The listing builds one solid part. Answer for the finished solid, in the listing's coordinates (mm). A direction names the side the tool comes from. Give positions to 0.01 mm unless a question says otherwise; leave off trailing zeros. Loops run counter-clockwise (first coordinate to the right, second up) from the corner with the lowest first, then second, coordinate; pieces in that order, holes last. Notation, with made-up numbers: (-8, 10.5) - (44, 10.5) arc R10 cw to (44, 22.5) - close; hole circle Ø10 at (-40, -21.5). An arc over 180 degrees is marked (long way). Write item = value, one per line. Start each with the question number.
1) The part is cut by section B-B on y = 30. State how many separate pieces and enclosed holes the cut face has, plus the area to 3 significant figures.
2) The part is cut by section C-C on x = 2.25. Write down the section's boundary in (y, z), plus the area to 3 significant figures.
3) Consider probe 1 along Z at (x, y) = (11.6, 0); probe 2 along X at (y, z) = (-15.5, 25); probe 3 along X at (y, z) = (-11, 26). Determine where each line is inside the solid, lowest interval first.
4) The mould has two halves that part along Z. Classify faces 1 (the conical face through (8.09, -25.76, 3.38)), 2 (the flat face through (14, -0.2, 10.4)), 3 (the flat face through (9, 5, -16)): +Z half, -Z half, draft (parallel to the pull), parting line (faces both ways), or undercut.
5) Flat-ended cylindrical pins translate along their axes: P1, Ø11.5, axis at y = 0, z = 0, coming from the +X side; P2, Ø1, axis at x = 1, y = 13, coming from the +Z side; P3, Ø3.5, axis at x = -0.5, y = 10.5, coming from the -Z side; P4, Ø12, axis at x = 3.5, z = 22, coming from the -Y side. Find the tip coordinate at first contact, or state that the pin passes through.
6) Which of the six approach directions +Z, -Z, +X, -X, +Y, -Y give full straight-line access (tool end or side, diameter ignored) to faces 4 (the flat face through (0, 11, -3)), 5 (the cylindrical face through (-6, 24.9, 5.5)), 6 (the flat face through (-9, 13, -12))?
7) The part is cut by section A-A on x = -6.75. Write down the section's boundary in (y, z), plus the area to 3 significant figures.
from build123d import *

# Parameters (mm, degrees)
CHAMFER1_SIZE      = 0.5
CHAMFER2_SIZE      = 0.5
FILLET2_R          = 1
CUT_EXTRUDE1_DEPTH = 58.484780595


with BuildPart() as part:
    # Sketch1 → Revolve1 (revolve)
    with BuildSketch(Plane(origin=(0, 0, 0), x_dir=(1, 0, 0), z_dir=(0, 1, 0))):
        Polygon((-14, 35.5), (-14, 23.5), (-9, 23.5), (-9, 16.5), (-14, 16.5), (-14, 9.5), (14, 9.5), (14, 16.5), (9, 16.5), (9, 23.5), (14, 23.5), (14, 35.5), (11, 35.5), (7.942693185, 25.5), (4.057306815, 25.5), (1, 35.5), (-1, 35.5), (-4.057306815, 25.5), (-7.942693185, 25.5), (-11, 35.5), align=None)
    revolve(axis=Axis((0, 0, 0), (-1, 0, 0)))

    # Chamfer1
    chamfer1_edges = [part.edges().sort_by_distance(p)[0] for p in [
        (14, 0, 9.5),
        (14, 0, 16.5),
        (14, 0, 35.5),
    ]]
    chamfer(chamfer1_edges, length=CHAMFER1_SIZE)

    # Chamfer2
    chamfer2_edges = [part.edges().sort_by_distance(p)[0] for p in [
        (-14, 0, 35.5),
        (-14, 0, 23.5),
        (-14, 0, 16.5),
        (-14, 0, 9.5),
    ]]
    chamfer(chamfer2_edges, length=CHAMFER2_SIZE)

    # Fillet2
    fillet2_edges = [part.edges().sort_by_distance(p)[0] for p in [
        (-9, 0, 23.5),
        (-9, 0, 16.5),
    ]]
    fillet(fillet2_edges, radius=FILLET2_R)

    # Sketch2 → Cut-Extrude1 (cut, through all)
    with BuildSketch(Plane(origin=(14, 0, 0), x_dir=(0, 0, -1), z_dir=(1, 0, 0))):
        Polygon((-3, 12.3), (-3, 7.432980878), (3, 7.432980878), (3, 9.5), (3, 12.3), align=None)
    extrude(amount=-CUT_EXTRUDE1_DEPTH, mode=Mode.SUBTRACT)


solid = part.part
Answer below:
q1.separate_pieces = 3
q1.enclosed_holes = 0
q1.area = 470 mm2
q2.outline = circle Ø62.82 at (0, 0); hole (9.01, -3) - (12.3, -3) - (12.3, 3) - (9.01, 3) arc R9.5 ccw (long way) to start
q2.area = 2,800 mm2
q3.probe_1 = -35.5 to -23.5, -16.5 to -9.5, 9.5 to 16.5, 23.5 to 35.5
q3.probe_2 = -14 to -9.14, -2.86 to 2.86, 9.14 to 14
q3.probe_3 = -14 to -8.78, -3.22 to 3.22, 8.78 to 14
q4.face_1 = parting line
q4.face_2 = draft
q4.face_3 = undercut
q5.P1 = through
q5.P2 = 33.23
q5.P3 = -34.4
q5.P4 = -31.41
q6.face_4 = +X, -X
q6.face_5 = none
q6.face_6 = -X
q7.outline = circle Ø51 at (0, 0); hole (9.01, -3) - (12.3, -3) - (12.3, 3) - (9.01, 3) arc R9.5 ccw (long way) to start
q7.area = 1,740 mm2
